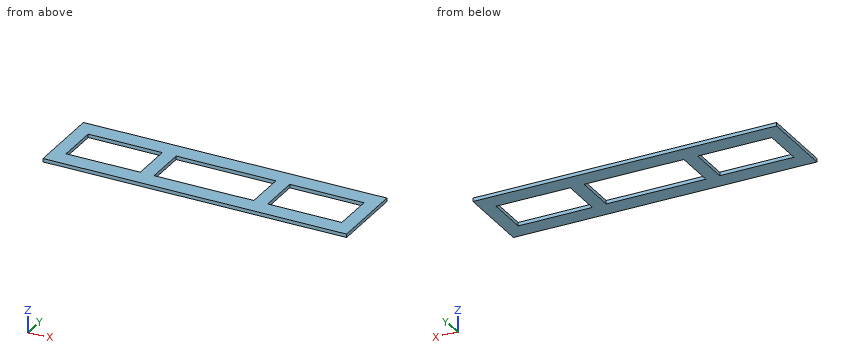
from build123d import *

# Parameters (mm, degrees)
F0_W     = 1663.7
F0_H     = 419.1
F0_W_2   = 406.4
F0_H_2   = 228.6
F0_W_3   = 546.1
F1_DEPTH = 19.05


with BuildPart() as f1:
    # F0 (on Top) → F1 (new body)
    with BuildSketch(Plane.XY):
        Rectangle(F0_W, F0_H)
        with Locations((-552.45, 0)):
            Rectangle(F0_W_2, F0_H_2, mode=Mode.SUBTRACT)
        Rectangle(F0_W_3, F0_H_2, mode=Mode.SUBTRACT)
        with Locations((552.45, 0)):
            Rectangle(F0_W_2, F0_H_2, mode=Mode.SUBTRACT)
    extrude(amount=F1_DEPTH)


solid = f1.part
Here's how the part is built. I have some questions about the finished solid (model axes, mm). Give positions to 0.01 mm unless a question says otherwise; leave off trailing zeros. Order: outer loops, then holes, each group sorted by start corner. A loop starts at its lowest first (then second) coordinate and runs counter-clockwise, first axis right, second up. Notation, with made-up numbers: M 47,43 L 87,43 A12 ccw 87,62 Z; hole C 7,-1 d8. An arc over 180 degrees is marked long. Answer as a JSON object with one key per item and string values. Group by question number.
1) Suppose I cut it at A-A, the plane y = 60.5. Write out the boundary of the cut face in (x, z), plus the area to 3 significant figures.
2) Please list where these lines run through material, in increasing order: L1, parallel to X at y = 91, z = 5.5; L2, parallel to Y at x = 127, z = 16.75. Write a range as [from, to].
3) Suppose I cut it at B-B, the plane z = 9. Write out the boundary of the cut face in (x, y), plus the area to 3 significant figures.
4) Suppose I cut it at C-C, the plane x = 527. Write out the boundary of the cut face in (y, z).
Results found:
{
 "1": {"outline": "M -831.85,0 L -755.65,0 L -755.65,19.05 L -831.85,19.05 Z; M -349.25,0 L -273.05,0 L -273.05,19.05 L -349.25,19.05 Z; M 273.05,0 L 349.25,0 L 349.25,19.05 L 273.05,19.05 Z; M 755.65,0 L 831.85,0 L 831.85,19.05 L 755.65,19.05 Z", "area": "5,810 mm²"},
 "2": {"L1": "[-831.85, -755.65], [-349.25, -273.05], [273.05, 349.25], [755.65, 831.85]", "L2": "[-209.55, -114.3], [114.3, 209.55]"},
 "3": {"outline": "M -831.85,-209.55 L 831.85,-209.55 L 831.85,209.55 L -831.85,209.55 Z; hole M -755.65,-114.3 L -349.25,-114.3 L -349.25,114.3 L -755.65,114.3 Z; hole M -273.05,-114.3 L 273.05,-114.3 L 273.05,114.3 L -273.05,114.3 Z; hole M 349.25,-114.3 L 755.65,-114.3 L 755.65,114.3 L 349.25,114.3 Z", "area": "387,000 mm²"},
 "4": {"outline": "M -209.55,0 L -114.3,0 L -114.3,19.05 L -209.55,19.05 Z; M 114.3,0 L 209.55,0 L 209.55,19.05 L 114.3,19.05 Z"}
}
